Can you work these out from the model? Positions are in its coordinate system, mm. A direction names the side the tool comes from. Give positions to 0.01 mm unless a question says otherwise; leave off trailing zeros. Write each loop counter-clockwise with the first axis right and the second up, starting at its lowest first coordinate (ties: lowest second). Pieces come first, ordered by that corner, then holes.
```python
from build123d import *

# Parameters (mm, degrees)
SKETCH_1_W      = 115
SKETCH_1_H      = 115
EXTRUDE_1_DEPTH = 3


with BuildPart() as part:
    # Эскиз1 → Бобышка-Вытянуть1 (new body)
    with BuildSketch(Plane(origin=(0, 0, 0), x_dir=(1, 0, 0), z_dir=(0, 1, 0))):
        Rectangle(SKETCH_1_W, SKETCH_1_H)
        with BuildLine():
            Line((-44.5, -52.5), (44.5, -52.5))
            ThreePointArc((44.5, -52.5), (50.156854249, -50.156854249), (52.5, -44.5))
            Line((52.5, -44.5), (52.5, 44.5))
            ThreePointArc((52.5, 44.5), (50.156854249, 50.156854249), (44.5, 52.5))
            Line((44.5, 52.5), (-44.5, 52.5))
            ThreePointArc((-44.5, 52.5), (-50.156854249, 50.156854249), (-52.5, 44.5))
            Line((-52.5, 44.5), (-52.5, -44.5))
            ThreePointArc((-52.5, -44.5), (-50.156854249, -50.156854249), (-44.5, -52.5))
        make_face(mode=Mode.SUBTRACT)
    extrude(amount=EXTRUDE_1_DEPTH)


solid = part.part
```
1) Suppose I cut it at A-A on z = -30. Write out the boundary of the cut face in (x, y).
Values follow:
outline: (-57.5, 0) - (-52.5, 0) - (-52.5, 3) - (-57.5, 3) - close; (52.5, 0) - (57.5, 0) - (57.5, 3) - (52.5, 3) - close
2) Suppose I cut it at C-C on y = 1.65. Write out the boundary of the cut face in (x, z).
Values follow:
outline: (-57.5, -57.5) - (57.5, -57.5) - (57.5, 57.5) - (-57.5, 57.5) - close; hole (-52.5, -44.5) arc R8 ccw to (-44.5, -52.5) - (44.5, -52.5) arc R8 ccw to (52.5, -44.5) - (52.5, 44.5) arc R8 ccw to (44.5, 52.5) - (-44.5, 52.5) arc R8 ccw to (-52.5, 44.5) - close
3) Please list where these lines run through material, in increasing order: L1, parallel to X at y = 1, z = 5; L2, parallel to X at y = 2.9, z = 49.5 (3 decimals).
Values follow:
L1: x = -57.5 to -52.5, 52.5 to 57.5
L2: x = -57.5 to -50.745, 50.745 to 57.5
4) For faces 1 (the face through (-57.5, 1, 1)), 2 (the face through (-50.094, 1.479, -50.219)), which set-ups out of +Z, -Z, +X, -X, +Y, -Y let a thin tool reach every point of the face, with its end or its side?
Values follow:
face 1: +Z, -Z, -X, +Y, -Y
face 2: +Y, -Y
5) If we mould it in two halves opening along Z, with no side actions, what happens to faces 3 (the face through (-1, 1, -57.5)), 4 (the face through (-1, 1, 57.5)), 5 (the face through (1, 1, -52.5)), 6 (the face through (0, 3, -56))? For each: +Z half, -Z half, draft (parallel to the pull), parting line (faces both ways), or undercut.
Values follow:
face 3: -Z half
face 4: +Z half
face 5: undercut
face 6: draft
6) Suppose I cut it at B-B on x = -30.5. Write out the boundary of the cut face in (y, z), plus the area to 3 significant figures.
Values follow:
outline: (0, -57.5) - (3, -57.5) - (3, -52.5) - (0, -52.5) - close; (0, 52.5) - (3, 52.5) - (3, 57.5) - (0, 57.5) - close
area: 30.0 mm2
